Solid Edge part; units mm, degrees
sketch "Sketch1" plane through (0, 0, 0) normal (0, 0, 1) x (1, 0, 0)
  line L0 (8.4135, 13.9146) -> (108.4135, 13.9146)
  line L1 (108.4135, 13.9146) -> (108.4135, 33.9146)
  line L2 (108.4135, 33.9146) -> (8.4135, 33.9146)
  line L3 (8.4135, 33.9146) -> (8.4135, 13.9146)
extrude "Protrusion1" add sketch "Sketch1" along normal blind 3
fillet "Round_1" radius 4 4 edges at (8.4135, 13.9146, 1.5) (108.4135, 13.9146, 1.5) (108.4135, 33.9146, 1.5) (8.4135, 33.9146, 1.5)
sketch "Sketch2" plane through (58.4135, 23.9146, 3) normal (0, 0, 1) x (1, 0, 0)
  circle A0 centre (-30, 0) radius 4
  circle A1 centre (0, 0) radius 4
  circle A2 centre (30, 0) radius 4
extrude "Cutout1" cut sketch "Sketch2" against normal through all
Geometry check sheet. Reference: the model listing, model coordinates, mm. Give positions to 0.01 mm unless a question says otherwise; leave off trailing zeros. Loops run counter-clockwise (first coordinate to the right, second up) from the corner with the lowest first, then second, coordinate; pieces in that order, holes last. Notation, with made-up numbers: (72, 79) - (130, 79) arc R21 ccw to (130, 108) - close; hole circle Ø4 at (-11.75, -13). An arc over 180 degrees is marked (long way). Use CSV: the item, a comma, the result in double quotes. Start each with the question number.
Q1. Section check D-D, the plane x = 57.5. Record the cut outline in (y, z).
Q2. Section check B-B, the plane x = 30. Record the cut outline in (y, z), and give its area (3 significant figures).
Q3. Section check C-C, the plane z = 1. Record the cut outline in (x, y).
Q4. Scan lines: probe 1 along X at (y, z) = (23.25, 0.45); probe 2 along X at (y, z) = (25, 2.9); probe 3 along Y at (x, z) = (88.5, 0.65). Record each from-to range of solid material in increasing order. Write a range as from..to.
Q5. Section check A-A, the plane y = 27. Record the cut outline in (x, z).
Q6. Release check for a two-part mould opening along Y. For faces 1 (the face through (108.414, 24, 1)), 2 (the face through (9.55, 15.12, 1.52)), 3 (the face through (62.229, 25.116, 1.521)) record: +Y half, -Y half, draft (parallel to the pull), parting line (faces both ways), or undercut.
Findings below:
1,outline,"(13.91, 0) - (20.02, 0) - (20.02, 3) - (13.91, 3) - close; (27.81, 0) - (33.91, 0) - (33.91, 3) - (27.81, 3) - close"
2,outline,"(13.91, 0) - (20.24, 0) - (20.24, 3) - (13.91, 3) - close; (27.59, 0) - (33.91, 0) - (33.91, 3) - (27.59, 3) - close"
2,area,"38.0 mm^2"
3,outline,"(8.41, 17.91) arc R4 ccw to (12.41, 13.91) - (104.41, 13.91) arc R4 ccw to (108.41, 17.91) - (108.41, 29.91) arc R4 ccw to (104.41, 33.91) - (12.41, 33.91) arc R4 ccw to (8.41, 29.91) - close; hole circle Ø8 at (28.41, 23.91); hole circle Ø8 at (58.41, 23.91); hole circle Ø8 at (88.41, 23.91)"
4,probe 1,"x = 8.41..24.47, 32.36..54.47, 62.36..84.47, 92.36..108.41"
4,probe 2,"x = 8.41..24.56, 32.26..54.56, 62.26..84.56, 92.26..108.41"
4,probe 3,"y = 13.91..19.92, 27.91..33.91"
5,outline,"(8.41, 0) - (25.87, 0) - (25.87, 3) - (8.41, 3) - close; (30.96, 0) - (55.87, 0) - (55.87, 3) - (30.96, 3) - close; (60.96, 0) - (85.87, 0) - (85.87, 3) - (60.96, 3) - close; (90.96, 0) - (108.41, 0) - (108.41, 3) - (90.96, 3) - close"
6,face 1,"draft"
6,face 2,"-Y half"
6,face 3,"undercut"
